CAD build for the part. Positions are in the model's coordinates, mm. Give positions to 0.01 mm unless a question says otherwise; leave off trailing zeros. Write each loop counter-clockwise with the first axis right and the second up, starting at its lowest first coordinate (ties: lowest second). Pieces come first, ordered by that corner, then holes. Notation, with made-up numbers: (4.25, 30) - (14.25, 30) arc R15 cw to (14.25, 39) - close; hole circle Ø7 at (88.5, -30.75). An arc over 180 degrees is marked (long way). Answer as a JSON object with one key per item and string values.
from build123d import *

# Parameters (mm, degrees)
BOSS_EXTRUDE1_DEPTH = 2
BOSS_EXTRUDE2_DEPTH = 1000
FILLET1_R           = 30


with BuildPart() as part:
    # Sketch1 → Boss-Extrude1 (new, symmetric)
    with BuildSketch(Plane.XY):
        Polygon((51.098896592, 549.111782584), (109.556303029, 650.722199952), (-190.085319823, 823.108777884), (-411.145086474, 1205.995525233), (-844.157788367, 955.995525233), (-622.202758989, 571.558137356), (-621.679381509, 229.965176242), (-501.679240657, 229.965176242), align=None)
    extrude(amount=BOSS_EXTRUDE1_DEPTH, both=True)

    # Sketch1_4 → Boss-Extrude2 (add, symmetric)
    with BuildSketch(Plane.XY):
        with BuildLine():
            ThreePointArc((-497.66471223, 873.157078986), (-512.30671881, 861.886187294), (-493.983532721, 859.502449096))
            Line((-493.983532721, 859.502449096), (-502.65143742, 864.489174287))
            Line((-502.65143742, 864.489174287), (-497.66471223, 873.157078986))
        make_face()
        with BuildLine():
            Line((-502.65143742, 864.489174287), (-493.983532721, 859.502449096))
            ThreePointArc((-493.983532721, 859.502449096), (-492.990199224, 861.908384387), (-492.65143742, 864.489174287))
            ThreePointArc((-492.65143742, 864.489174287), (-493.995016338, 869.495807292), (-497.66471223, 873.157078986))
            Line((-497.66471223, 873.157078986), (-502.65143742, 864.489174287))
        make_face()
    extrude(amount=BOSS_EXTRUDE2_DEPTH, both=True)

    # Fillet1
    fillet1_edges = [part.edges().sort_by_distance(p)[0] for p in [
        (-621.679381509, 229.965176242, 0),
        (-622.202758989, 571.558137356, 0),
        (-844.157788367, 955.995525233, 0),
        (-411.145086474, 1205.995525233, 0),
        (-190.085319823, 823.108777884, 0),
        (109.556303029, 650.722199952, 0),
    ]]
    fillet(fillet1_edges, radius=FILLET1_R)


solid = part.part
Item 1: Cut at B-B (y = 1024.5). Give the cut face in (x, z).
Entries:
{"outline": "(-725.5, -2) - (-306.36, -2) - (-306.36, 2) - (-725.5, 2) - close"}
Item 2: Probe line 1 (Z direction, x = -112.5, y = 750). List the from-to ranges inside material, lowest first. Write a range as from..to.
Entries:
{"line 1": "-2..2"}
Item 3: Cut at A-A (z = -507.5). Give the cut face in (x, y), and give its area (3 significant figures).
Entries:
{"outline": "circle Ø20 at (-502.65, 864.49)", "area": "314 mm2"}
Item 4: Flat gauge pins, fed straight in: P1, Ø3, axis at x = -526.5, y = 561, coming from the +Z side; P2, Ø4, axis at x = -417.5, y = 508, coming from the -Z side. Where does each tip first touch, or does it go through?
Entries:
{"P1": "z = 2", "P2": "z = -2"}
Item 5: Cut at C-C (x = -283.5). Give the cut face in (y, z), and give its area (3 significant figures).
Entries:
{"outline": "(355.93, -2) - (984.91, -2) - (984.91, 2) - (355.93, 2) - close", "area": "2,520 mm2"}
